Geometry check sheet. Reference: the model listing, model coordinates, mm. Face numbers are marked on the shaded views. A direction names the side the tool comes from. Give positions to 0.01 mm unless a question says otherwise; leave off trailing zeros. Write each loop counter-clockwise with the first axis right and the second up, starting at its lowest first coordinate (ties: lowest second). Pieces come first, ordered by that corner, then holes.
(1) Mould release check, pull along X, two halves, no side actions. Record for the marked faces 1, 2 and 3: +X half, -X half, draft (parallel to the pull), parting line (faces both ways), or undercut.
(2) Thickness scan on line 1 along Z through (x, y) = (-4, -5.5); line 2 along Z through (x, y) = (-34, -16.75); line 3 along X through (y, z) = (-9.25, 7.5). Record the ranges inside material, lowest first.
(3) Tool access check on the marked faces 4, 5 and 6. Record the directions out of +Z, -Z, +X, -X, +Y, -Y that give a thin tool (end or side, any length) a straight path to the whole face; none if there is none.
(4) Cross-section at A-A (z = 13.5). Record the boundary of the cut face in (x, y).
(5) Cross-section at B-B (y = -10.5). Record the boundary of the cut face in (x, z).
(6) Depth check by flat-ended pin: P1, Ø12, axis at x = -1.5, y = -13.5, coming from the -Z side; P2, Ø5, axis at x = -18, y = -18.5, coming from the -Z side; P3, Ø12, axis at x = 15.5, y = -12, coming from the -Z side; P4, Ø5, axis at x = -9, z = 0.5, coming from the +Y side. Enter the tip coordinate at first touch or a pass-through.
(7) Cross-section at C-C (x = 4). Record the boundary of the cut face in (y, z), and give its area (3 significant figures).
(8) Cross-section at D-D (z = -11.5). Record the boundary of the cut face in (x, y), and give its area (3 significant figures).
```python
from build123d import *

# Parameters (mm, degrees)
F0_W     = 15.156722
F0_H     = 16.031148
F1_DEPTH = 25.4
F2_DEPTH = 25.4
F3_DEPTH = 25.4


with BuildPart() as f1:
    # F0 (on Front) → F1 (new body)
    with BuildSketch(Plane.XZ):
        Rectangle(F0_W, F0_H)
        Polygon((7.578361, 8.015574), (7.578361, -8.015574), (37.891805, -17.634263), (38.766231, 16.468361), align=None)
        Polygon((-45.761641, -16.176885), (-7.578361, -8.015574), (-7.578361, 8.015574), (-45.761641, 16.468361), align=None)
    extrude(amount=F1_DEPTH)

    # F0 (on Front) → F2 (join)
    with BuildSketch(Plane.XZ):
        Rectangle(F0_W, F0_H)
        Polygon((7.578361, 8.015574), (7.578361, -8.015574), (37.891805, -17.634263), (38.766231, 16.468361), align=None)
        Polygon((-45.761641, -16.176885), (-7.578361, -8.015574), (-7.578361, 8.015574), (-45.761641, 16.468361), align=None)
    extrude(amount=F2_DEPTH)

    # F0 (on Front) → F3 (join)
    with BuildSketch(Plane.XZ):
        Rectangle(F0_W, F0_H)
        Polygon((7.578361, 8.015574), (7.578361, -8.015574), (37.891805, -17.634263), (38.766231, 16.468361), align=None)
        Polygon((-45.761641, -16.176885), (-7.578361, -8.015574), (-7.578361, 8.015574), (-45.761641, 16.468361), align=None)
    extrude(amount=F3_DEPTH)


solid = f1.part
```
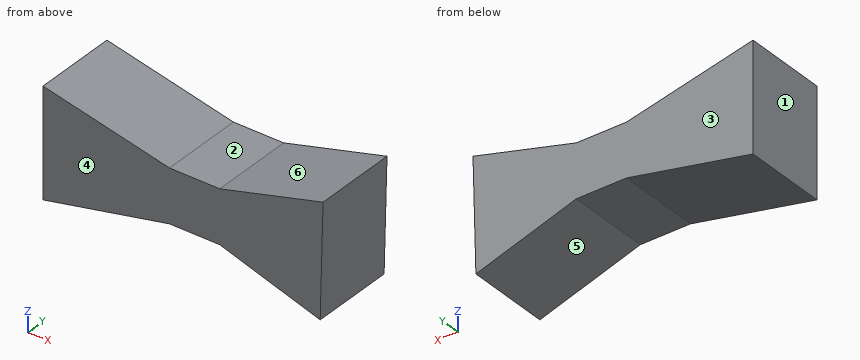
Reply:
1. face 1: -X half
1. face 2: undercut
1. face 3: draft
2. line 1: z = -8.02 to 8.02
2. line 2: z = -13.66 to 13.86
2. line 3: x = -45.76 to 38.54
3. face 4: +Z, -Z, +X, -X, -Y
3. face 5: -Z, +Y, -Y
3. face 6: +Z, +Y, -Y
4. outline: (-45.76, -25.4) - (-32.35, -25.4) - (-32.35, 0) - (-45.76, 0) - close; (27.81, -25.4) - (38.69, -25.4) - (38.69, 0) - (27.81, 0) - close
5. outline: (-45.76, -16.18) - (-7.58, -8.02) - (7.58, -8.02) - (37.89, -17.63) - (38.77, 16.47) - (7.58, 8.02) - (-7.58, 8.02) - (-45.76, 16.47) - close
6. P1: stops at z = -8.02
6. P2: stops at z = -10.78
6. P3: stops at z = -12.43
6. P4: stops at y = 0
7. outline: (-25.4, -8.02) - (0, -8.02) - (0, 8.02) - (-25.4, 8.02) - close
7. area: 407 mm2
8. outline: (-45.76, -25.4) - (-23.88, -25.4) - (-23.88, 0) - (-45.76, 0) - close; (18.56, -25.4) - (38.05, -25.4) - (38.05, 0) - (18.56, 0) - close
8. area: 1,050 mm2
